from build123d import *

# Parameters (mm, degrees)
F2_DEPTH = 3
F3_DEPTH = 3


with BuildPart() as f2:
    # F0 (on Front) → F2 (new body)
    with BuildSketch(Plane.XZ):
        with BuildLine():
            Line((0, 110), (-37.1250543006, 110))
            ThreePointArc((-37.1250543006, 110), (-57.0530283082, 108.1392327186), (-76.2920156121, 102.6212647557))
            ThreePointArc((-76.2920156121, 102.6212647557), (-107.8053845023, 88.0195194413), (-137.2898370028, 69.6627646685))
            ThreePointArc((-137.2898370028, 69.6627646685), (-168.2962814604, 45.2722513622), (-196.811914444, 18.0113743991))
            ThreePointArc((-196.811914444, 18.0113743991), (-198.6562382919, 5.922529929), (-187.9573911428, 0))
            ThreePointArc((-187.9573911428, 0), (-172.1749520727, 3.7961120216), (-157.950386405, 11.6164432839))
            ThreePointArc((-157.950386405, 11.6164432839), (-133.5467802063, 29.7456036712), (-109.2505156994, 48.0183698237))
            ThreePointArc((-109.2505156994, 48.0183698237), (-94.8181161846, 56.7914277787), (-78.9122924344, 62.4716982356))
            ThreePointArc((-78.9122924344, 62.4716982356), (-62.1941450585, 65.5321609692), (-45.2291222508, 66.5572877705))
            Line((-45.2291222508, 66.5572877705), (0, 66.5572877705))
            Line((0, 66.5572877705), (45.2291222508, 66.5572877705))
            ThreePointArc((45.2291222508, 66.5572877705), (62.1941450585, 65.5321609692), (78.9122924344, 62.4716982356))
            ThreePointArc((78.9122924344, 62.4716982356), (94.8181161846, 56.7914277787), (109.2505156994, 48.0183698237))
            ThreePointArc((109.2505156994, 48.0183698237), (133.5467802063, 29.7456036712), (157.950386405, 11.6164432839))
            ThreePointArc((157.950386405, 11.6164432839), (172.1749520727, 3.7961120216), (187.9573911428, 0))
            ThreePointArc((187.9573911428, 0), (198.6562382919, 5.922529929), (196.811914444, 18.0113743991))
            ThreePointArc((196.811914444, 18.0113743991), (168.2962814604, 45.2722513622), (137.2898370028, 69.6627646685))
            ThreePointArc((137.2898370028, 69.6627646685), (107.8053845023, 88.0195194413), (76.2920156121, 102.6212647557))
            ThreePointArc((76.2920156121, 102.6212647557), (57.0530283082, 108.1392327186), (37.1250543006, 110))
            Line((37.1250543006, 110), (0, 110))
        make_face()
    extrude(amount=F2_DEPTH)

    # F1 (on Front) → F3 (join)
    with BuildSketch(Plane.XZ):
        with BuildLine():
            ThreePointArc((18.8345826463, 158.9782924416), (19.1860958712, 215.6277740938), (-37.2, 221.0954541697))
            Line((-37.2, 221.0954541697), (-46.0592777571, 214.4509958519))
            ThreePointArc((-46.0592777571, 214.4509958519), (-49.9587726937, 207.8652094143), (-48.0592777571, 200.4509958519))
            Line((-48.0592777571, 200.4509958519), (-45.0592777571, 196.4509958519))
            ThreePointArc((-45.0592777571, 196.4509958519), (-41.7663845383, 194.5012483836), (-38.0592777571, 195.4509958519))
            Line((-38.0592777571, 195.4509958519), (-25.2, 205.0954541697))
            ThreePointArc((-25.2, 205.0954541697), (5.6, 200.6954541697), (1.2, 169.8954541697))
            ThreePointArc((1.2, 169.8954541697), (-5.571825393, 161.7813668662), (-8, 151.4954541697))
            Line((-8, 151.4954541697), (-8, 110))
            Line((-8, 110), (0, 110))
            Line((0, 110), (12, 110))
            Line((12, 110), (12, 151.4954541697))
            ThreePointArc((12, 151.4954541697), (12.316718427, 152.8370949562), (13.2, 153.8954541697))
            ThreePointArc((13.2, 153.8954541697), (15.3055154559, 155.5829358472), (17.2983292582, 157.4021342685))
            add(Edge.make_bspline(
                [(18.8345826463, 158.9782924416), (18.2685657224, 158.4677005018), (17.7583091445, 157.9420185701), (17.2983292582, 157.4021342685)],
                knots=[0, 0, 0, 0, 0.0332714109, 0.0332714109, 0.0332714109, 0.0332714109], degree=3))
        make_face()
        with BuildLine():
            ThreePointArc((17.2983292582, 157.4021342685), (18.0767824439, 158.180148307), (18.8345826463, 158.9782924416))
            add(Edge.make_bspline(
                [(18.8345826463, 158.9782924416), (18.2685657224, 158.4677005018), (17.7583091445, 157.9420185701), (17.2983292582, 157.4021342685)],
                knots=[0, 0, 0, 0, 0.0332714109, 0.0332714109, 0.0332714109, 0.0332714109], degree=3))
        make_face()
        with BuildLine():
            add(Edge.make_bspline(
                [(17.2983292582, 157.4021342685), (13.1793035086, 152.5675808311), (12.9884623094, 139.527426253), (13.3703276725, 116.5931182655), (29.7821242027, 110), (33.8129806474, 110)],
                knots=[0.0332714109, 0.0332714109, 0.0332714109, 0.0332714109, 0.3312100872, 0.6836806519, 1, 1, 1, 1], degree=3))
            ThreePointArc((17.2983292582, 157.4021342685), (15.3055154559, 155.5829358472), (13.2, 153.8954541697))
            ThreePointArc((13.2, 153.8954541697), (12.316718427, 152.8370949562), (12, 151.4954541697))
            Line((12, 151.4954541697), (12, 110))
            Line((12, 110), (33.8129806474, 110))
        make_face()
        with BuildLine():
            ThreePointArc((-8, 151.4954541697), (-5.571825393, 161.7813668662), (1.2, 169.8954541697))
            add(Edge.make_bspline(
                [(-36.0568419915, 110), (-19.4195834096, 110), (-18.0177646467, 138.2709232819), (-12.939977235, 158.3678372994), (-4.7115848759, 166.2572265506), (1.2, 169.8954541697)],
                knots=[0, 0, 0, 0, 0.3938915377, 0.7136667849, 1, 1, 1, 1], degree=3))
            Line((-36.0568419915, 110), (-8, 110))
            Line((-8, 110), (-8, 151.4954541697))
        make_face()
    extrude(amount=F3_DEPTH)


solid = f2.part
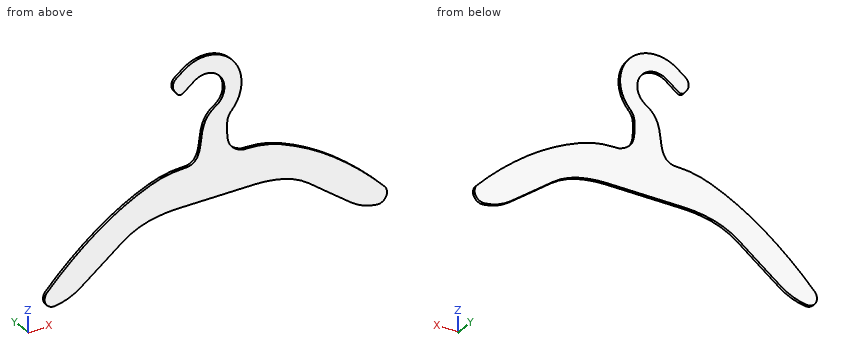
Here's how the part is built. I have some questions about the finished solid (model axes, mm). Coordinates: 2 decimals unless noted, no trailing zeros. Order: outer loops, then holes, each group sorted by start corner. A loop starts at its lowest first (then second) coordinate and runs counter-clockwise, first axis right, second up. Notation, with made-up numbers: M 85,74.25 L 133,74.25 A27 ccw 133,112.25 Z; hole C 6,32 d3. An arc over 180 degrees is marked long. Answer as CSV lines item,"result". Start each with the question number.
1. I want a section at C-C, the plane x = -142.5. Write out the boundary of the cut face in (y, z).
2. I need wall thicknesses on line 1 (Z direction, x = -45.5, y = -2.25); line 2 (Z direction, x = -28.5, y = -0.7); line 3 (X direction, y = -2.1, z = 187.5). Which ranges of each line are inside material? Lowest first, please. Write a range as [from, to].
3. For pin 1 (3 mm diameter, centred on x = 9.5, z = 153.5, fed in from +Y); pin 2 (0.5 mm diameter, centred on x = -36.5, y = -2, fed in from +Z); pin 3 (1.5 mm diameter, centred on y = -0.5, z = 46.5, fed in from -X); pin 4 (1 mm diameter, centred on y = -0.5, z = 60, fed in from -X), each with a flat end and sliding along its axis, tell me the tip position at first contact or that it passes through.
4. I want a section at A-A, the plane z = 58. Write out the boundary of the cut face in (x, y), and give its area (3 significant figures).
5. I want a section at B-B, the plane x = -85.5. Write out the boundary of the cut face in (y, z), and give its area (3 significant figures).
Recorded:
1,outline,"M -3,23.07 L 0,23.07 L 0,65.89 L -3,65.89 Z"
2,line 1,"z = [66.56, 109.67], [197.04, 214.87]"
2,line 2,"z = [66.56, 111.41], [202.62, 226.12]"
2,line 3,"x = [10, 30]"
3,pin 1,"stops at y = 0"
3,pin 2,"stops at z = 221.79"
3,pin 3,"stops at x = -167.74"
3,pin 4,"stops at x = -150.96"
4,outline,"M -152.88,-3 L -92.16,-3 L -92.16,0 L -152.88,0 Z; M 92.16,-3 L 152.88,-3 L 152.88,0 L 92.16,0 Z"
4,area,"364 mm2"
5,outline,"M -3,60.56 L 0,60.56 L 0,98.84 L -3,98.84 Z"
5,area,"115 mm2"
